from build123d import *

# Parameters (mm, degrees)
F1_DEPTH = 311.15
F2_T     = -7.62


# Not quite as in the source:
# - a feature names something its author has since deleted; it is built from what else it names


with BuildPart() as f1:
    # F0 (on Top) → F1 (new body)
    with BuildSketch(Plane.XY):
        Polygon((342.2408003828, -255.094484383), (342.2408003828, 173.456788063), (-254.6591996172, 173.456788063), (-254.6591996172, -197.8495568037), (-254.6591996172, -255.094484383), (334.2911142349, -255.094484383), align=None)
    extrude(amount=F1_DEPTH)

    # F2
    f2_openings = [f1.faces().sort_by_distance(p)[0] for p in [
        (43.7908, -40.818848, 311.15),
    ]]
    offset(amount=F2_T, openings=f2_openings)


solid = f1.part
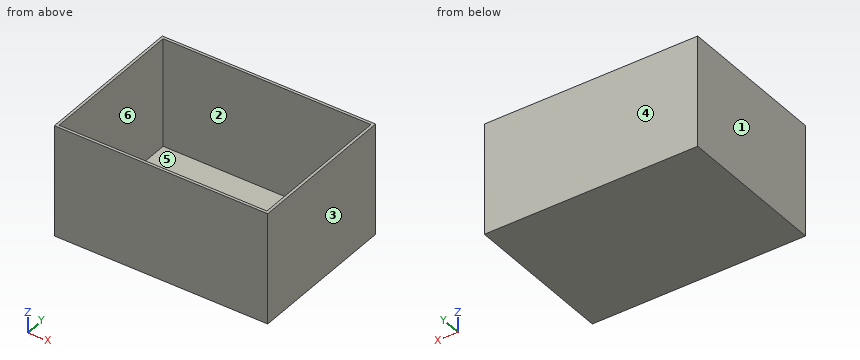
Could you check a few things on this model? Use its own coordinates, in mm. Face numbers are marked on the shaded views. A direction names the side the tool comes from. Round coordinates to 2 decimals unless told otherwise and drop trailing zeros. Write each loop counter-clockwise with the first axis right and the second up, starting at its lowest first coordinate (ties: lowest second). Pieces come first, ordered by that corner, then holes. Notation, with made-up numbers: (78, 82.25) - (115, 82.25) arc R27 cw to (115, 112.25) - close; hole circle Ø3 at (71.25, 17.5). An arc over 180 degrees is marked (long way). Put each result on its own line as item: value. Start each with the question number.
(1) I want a section at C-C, the plane x = 90. Please give me the cut outline in (y, z).
(2) I need wall thicknesses on probe 1 along Y at (x, z) = (104, 222.5); probe 2 along X at (y, z) = (-36, 265); probe 3 along Z at (x, y) = (275, 26). Which ranges of each line are inside material? Lowest first, please.
(3) Thinking about a two-plate mould opening in X: for the marked faces 3, 4, 5 and 6, which applies, released by +X, released by -X, zero draft, split by the parting line, or undercut?
(4) For the marked faces 1 and 2, which set-ups out of +Z, -Z, +X, -X, +Y, -Y let a thin tool reach every point of the face, with its end or its side?
(5) I want a section at A-A, the plane z = 249.5. Please give me the cut outline in (x, y), plus the area to 3 significant figures.
(6) I want a section at B-B, the plane y = -107. Please give me the cut outline in (x, z).
Here are the results:
1. outline: (-255.09, 0) - (173.46, 0) - (173.46, 311.15) - (165.84, 311.15) - (165.84, 7.62) - (-247.47, 7.62) - (-247.47, 311.15) - (-255.09, 311.15) - close
2. probe 1: y = -255.09 to -247.47, 165.84 to 173.46
2. probe 2: x = -254.66 to -247.04, 334.62 to 342.24
2. probe 3: z = 0 to 7.62
3. face 3: released by +X
3. face 4: zero draft
3. face 5: undercut
3. face 6: undercut
4. face 1: +Z, -Z, -X, +Y, -Y
4. face 2: +Z
5. outline: (-254.66, -255.09) - (342.24, -255.09) - (342.24, 173.46) - (-254.66, 173.46) - close; hole (-247.04, -247.47) - (334.62, -247.47) - (334.62, 165.84) - (-247.04, 165.84) - close
5. area: 15,400 mm^2
6. outline: (-254.66, 0) - (342.24, 0) - (342.24, 311.15) - (334.62, 311.15) - (334.62, 7.62) - (-247.04, 7.62) - (-247.04, 311.15) - (-254.66, 311.15) - close
